Input: part model. Units: mm. Frame: model coordinates. Face numbers are marked on the shaded views. A direction names the side the tool comes from. Give positions to 0.01 mm unless a question says otherwise; leave off trailing zeros. Loops run counter-clockwise (first coordinate to the right, second up) from the corner with the lowest first, then second, coordinate; pieces in that order, holes last. Notation, with made-up numbers: (56, 77.25) - (77, 77.25) arc R11 ccw to (77, 87.25) - close; hole circle Ø4 at (43, 33.25). An arc over 180 degrees is marked (long way). One line per item, written item: value.
Autodesk Inventor part; units mm, degrees
ref_plane "YZ Plane" through (0, 0, 0) normal (1, 0, 0) x (0, 1, 0)
ref_plane "XZ Plane" through (0, 0, 0) normal (0, 1, 0) x (-1, 0, 0)
ref_plane "XY Plane" through (0, 0, 0) normal (0, 0, 1) x (1, 0, 0)
sketch "Sketch1" plane through (0, 0, 0) normal (0, 0, 1) x (1, 0, 0)
  line L0 (5, 9.798) -> (5, -9.798)
  line L1 (-5, -9.798) -> (-5, 9.798)
  arc A0 (-5, -9.798) -> (5, -9.798) centre (0, 0) ccw
  arc A1 (5, 9.798) -> (-5, 9.798) centre (0, 0) ccw
  point P0 (0, 12.4867)
  point P1 (5, 0)
  dimension "d1" = 10
  dimension "d2" = 11
  dimension "d3" = 11
  dimension "d4" = 5
  dimension "d5" = 12.4867
extrude "Extrusion1" add sketch "Sketch1" along normal blind 22
chamfer "Chamfer1" distance 0.5 angle 45 12 edges at (0, 11, 22) (5, 0, 22) (0, -11, 22) (-5, 0, 22) (5, 9.798, 11) (-5, 9.798, 11) (0, 11, 0) (5, 0, 0) (5, -9.798, 11) (0, -11, 0) (-5, 0, 0) (-5, -9.798, 11)
sketch "Sketch2" plane through (0, 0, 22) normal (0, 0, 1) x (1, 0, 0)
  arc A0 (4.5, 9.4868) -> (-4.5, 9.4868) centre (0, 0) ccw
hole "Hole1" at (0, 0, 22) direction (0, 0, -1) diameter 4.134 depth 8
sketch "Sketch3" plane through (5, -9.298, 0.5) normal (1, 0, 0) x (0, 0, -1)
  line L0 (-21, 18.5959) -> (0, 18.5959)
  line L1 (-21, 0) -> (-21, 18.5959)
  point P0 (0.5, 9.298)
  point P1 (-10.5, 9.298)
  point P2 (-21, 9.298)
  point P3 (-10.5, 18.5959)
hole "Hole2" at (5, 0, 11) direction (-1, 0, 0) diameter 6.5 end through all
properties part number "19 - Crosshead" material "Bronze, Soft Tin"
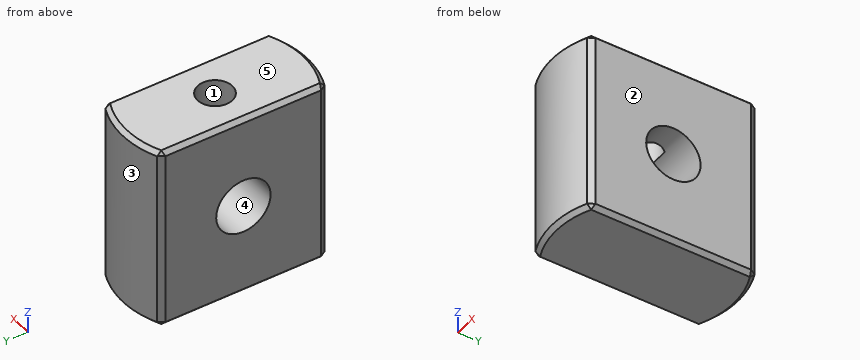
Item 1: Section B-B, the plane z = 16.75. Output: boundary loops of the cut face in (x, y), and give its area (3 significant figures).
Verdict:
outline: (-5, -9.3) - (-4.55, -10.02) arc R11 ccw to (4.55, -10.02) - (5, -9.3) - (5, 9.3) - (4.55, 10.02) arc R11 ccw to (-4.55, 10.02) - (-5, 9.3) - close; hole circle Ø4.13 at (0, 0)
area: 198 mm^2
Item 2: Section D-D, the plane x = 0. Output: boundary loops of the cut face in (y, z).
Verdict:
outline: (-11, 0.5) - (-10.5, 0) - (10.5, 0) - (11, 0.5) - (11, 21.5) - (10.5, 22) - (2.07, 22) - (2.07, 14) - (1.25, 14) arc R3.25 cw (long way) to (-1.25, 14) - (-2.07, 14) - (-2.07, 22) - (-10.5, 22) - (-11, 21.5) - close
Item 3: Section A-A, the plane y = 0. Output: boundary loops of the cut face in (x, z), and give its area (3 significant figures).
Verdict:
outline: (-5, 0.5) - (-4.5, 0) - (4.5, 0) - (5, 0.5) - (5, 7.75) - (-5, 7.75) - close; (-5, 14.25) - (-2.07, 14.25) - (-2.07, 22) - (-4.5, 22) - (-5, 21.5) - close; (2.07, 14.25) - (5, 14.25) - (5, 21.5) - (4.5, 22) - (2.07, 22) - close
area: 122 mm^2
Item 4: Material intervals for L1, parallel to Y at x = 0, z = 16.5; L2, parallel to X at y = 0, z = 16.25; L3, parallel to Z at x = 1, y = 0, sorted ascending.
Verdict:
L1: y = -11 to -2.07, 2.07 to 11
L2: x = -5 to -2.07, 2.07 to 5
L3: z = 0 to 7.75
Item 5: Section C-C, the plane z = 11. Output: boundary loops of the cut face in (x, y), and give its area (3 significant figures).
Verdict:
outline: (-5, -9.3) - (-4.55, -10.02) arc R11 ccw to (4.55, -10.02) - (5, -9.3) - (5, -3.25) - (-5, -3.25) - close; (-5, 3.25) - (5, 3.25) - (5, 9.3) - (4.55, 10.02) arc R11 ccw to (-4.55, 10.02) - (-5, 9.3) - close
area: 147 mm^2
Item 6: Draft query along Y for the marked faces 3, 4 and 5. Return one class per face: pulls with the +Y half, pulls with the -Y half, needs draft (parallel to the pull), parting line crosses it, or undercut.
Verdict:
face 3: pulls with the +Y half
face 4: undercut
face 5: needs draft
Item 7: Pin query (flat end, axial travel): P1, Ø1.5, axis at x = 1.5, z = 2.5, coming from the -Y side. Return the tip coordinate at first contact, or that it passes through.
Verdict:
P1: stops at y = -10.97
Item 8: Access query for the marked faces 1 and 2. Directions: +Z, -Z, +X, -X, +Y, -Y. A direction counts if a zero-diameter tool reaches every point of the face in a straight line with its end or side. Return the directions, or none.
Verdict:
face 1: +Z
face 2: +Z, -Z, +X, +Y, -Y
